Autodesk Inventor part; units mm, degrees
ref_plane "РабПлоскость1" through (18, -5, 16.3) normal (0, 0, -1) x (-1, 0, 0)
ref_plane "YZ Plane" through (0, 0, 0) normal (1, 0, 0) x (0, 1, 0)
ref_plane "XZ Plane" through (0, 0, 0) normal (0, 1, 0) x (-1, 0, 0)
sketch "Эскиз2" plane through (0, 0, 0) normal (1, 0, 0) x (0, 1, 0)
  line L0 (0, 0) -> (-20.5, 0)
  line L1 (-20.5, 0) -> (-20.5, 32.6)
  line L2 (-20.5, 32.6) -> (0, 32.6)
  line L3 (0, 32.6) -> (0, 0)
  line L4 (-20.5, 0) -> (-20.5, 7)
  line L5 (-20.5, 7) -> (-5, 7)
  line L6 (-5, 7) -> (-5, 25.6)
  line L7 (-5, 25.6) -> (-20.5, 25.6)
  line L8 (-20.5, 25.6) -> (-20.5, 7)
  point P0 (0, 3)
  dimension "d0" = 20.5
  dimension "d1" = 32.6
  dimension "d2" = 7
  dimension "d3" = 15.5
  dimension "d4" = 18.6
extrude "Выдавливание1" add sketch "Эскиз2" along normal blind 18 contours L0 L1 L5 L6 L7 L2 L3
sketch "Эскиз4" plane through (0, -20.5, 32.6) normal (0, 0, 1) x (1, 0, 0)
  line L0 (0, 0) -> (18, 0)
  line L1 (9, 0) -> (9, 7)
  circle A0 centre (9, 7) radius 4
  point P0 (0, 20.5)
  dimension "d7" = 7
  dimension "d8" = 8
extrude "Выдавливание2" cut sketch "Эскиз4" along normal blind 3 from surface at -7
ref_plane "РабПлоскость1" through (18, -5, 16.3) normal (0, 0, -1) x (-1, 0, 0)
mirror "Зеркальное отражение1" about plane through (18, -5, 16.3) normal (0, 0, -1) of "Выдавливание2"
sketch "Эскиз6" plane through (0, -20.5, 32.6) normal (0, 0, 1) x (1, 0, 0)
  circle A0 centre (9, 7) radius 4
  circle A1 centre (9, 7) radius 2.25
  point P0 (0, 20.5)
  dimension "d11" = 4.5
extrude "Выдавливание3" cut sketch "Эскиз6" against normal through all contours A1
fillet "Сопряжение1" radius 9 4 edges at (18, -20.5, 29.1) (0, -20.5, 29.1) (18, -20.5, 3.5) (0, -20.5, 3.5)
equation "\"d2\" = -0.5 * d4 + 0.5 * d1"
properties part number "Крепление кулака"
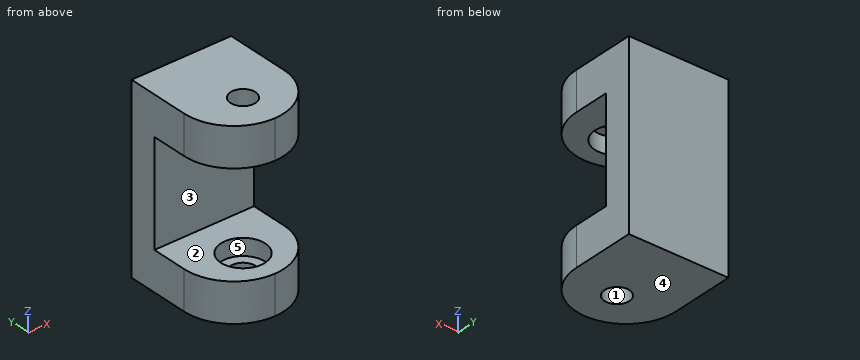
Source: CAD feature listing. Evaluate the final solid. Frame: model axes, mm. Face numbers are marked on the shaded views. A direction names the side the tool comes from. Give positions to 0.01 mm unless a question says otherwise; leave off trailing zeros. Write each loop counter-clockwise with the first axis right and the second up, starting at its lowest first coordinate (ties: lowest second). Pieces come first, ordered by that corner, then holes. Notation, with made-up numbers: M 59,39.5 L 98,39.5 A25 cw 98,71.5 Z; hole C -39.5,4 d2. An arc over 180 degrees is marked long. Return JSON: item names as keys, results as strings. Group by question number.
1) Set-up query: the marked faces 1 and 2. Return all of +Z, -Z, +X, -X, +Y, -Y with unobstructed straight access to the full face (end or side cutting, diameter ignored); none if empty.
2) Draft query along Y for the marked faces 3, 4 and 5. Return one class per face: released by +Y, released by -Y, zero draft, split by the parting line, or undercut.
3) Ray query, L1, parallel to Z at x = 6.25, y = -16.5; L2, parallel to Y at x = 9, z = 31.45; L3, parallel to Z at x = 5.75, y = -14.25. Return the intervals inside material, ascending.
4) Cut plane D-D, the plane x = 7.25. Output: boundary loops of the cut face in (y, z).
5) Cut plane C-C, the plane y = -13.5. Output: boundary loops of the cut face in (x, z).
6) First-contact query: pin 1 Ø1.5 at (x, z) = (2.5, 11.5) entering from -Y; pin 2 Ø2 at (x, y) = (8, -13.5) entering from -Z; pin 3 Ø5 at (y, z) = (-15.5, 6.5) entering from +X. Flat tips, straight axial feed; report the tip coordinate or a pass-through.
7) Cut plane A-A, the plane y = -7. Output: boundary loops of the cut face in (x, z).
Data:
{
 "1": {"face 1": "+Z, -Z", "face 2": "+X, -X, -Y"},
 "2": {"face 3": "released by -Y", "face 4": "zero draft", "face 5": "undercut"},
 "3": {"L1": "z = 0 to 7, 25.6 to 32.6", "L2": "y = -20.5 to -15.75, -11.25 to 0", "L3": "z = 0 to 4, 28.6 to 32.6"},
 "4": {"outline": "M -20.33,0 L -14.91,0 L -14.91,4 L -17.1,4 L -17.1,7 L -20.33,7 Z; M -20.33,25.6 L -17.1,25.6 L -17.1,28.6 L -14.91,28.6 L -14.91,32.6 L -20.33,32.6 Z; M -12.09,0 L 0,0 L 0,32.6 L -12.09,32.6 L -12.09,28.6 L -9.9,28.6 L -9.9,25.6 L -5,25.6 L -5,7 L -9.9,7 L -9.9,4 L -12.09,4 Z"},
 "5": {"outline": "M 0.23,0 L 6.75,0 L 6.75,4 L 5,4 L 5,7 L 0.23,7 Z; M 0.23,25.6 L 5,25.6 L 5,28.6 L 6.75,28.6 L 6.75,32.6 L 0.23,32.6 Z; M 11.25,0 L 17.77,0 L 17.77,7 L 13,7 L 13,4 L 11.25,4 Z; M 11.25,28.6 L 13,28.6 L 13,25.6 L 17.77,25.6 L 17.77,32.6 L 11.25,32.6 Z"},
 "6": {"pin 1": "stops at y = -5", "pin 2": "passes through", "pin 3": "stops at x = 17.87"},
 "7": {"outline": "M 0,0 L 18,0 L 18,7 L 0,7 Z; M 0,25.6 L 18,25.6 L 18,32.6 L 0,32.6 Z"}
}
